```python
from build123d import *

# Parameters (mm, degrees)
F0_R     = 25
F1_DEPTH = 50
F2_R     = 25.5
F3_DEPTH = 10
F4_R     = 2
F5_R     = 1


with BuildPart() as f1:
    # F0 (on Top) → F1 (new body)
    with BuildSketch(Plane.XY):
        Circle(F0_R)
    extrude(amount=F1_DEPTH)

    # F2 (on face) → F3 (join)
    with BuildSketch(Plane.XY.offset(50)):
        Circle(F2_R)
    extrude(amount=F3_DEPTH)

    # F4
    f4_edges = [f1.edges().sort_by_distance(p)[0] for p in [
        (-25.5, 0, 60),
    ]]
    fillet(f4_edges, radius=F4_R)

    # F5
    f5_edges = [f1.edges().sort_by_distance(p)[0] for p in [
        (-25, 0, 0),
    ]]
    fillet(f5_edges, radius=F5_R)


solid = f1.part
```
The listing builds one solid part. Answer for the finished solid, in the listing's coordinates (mm). A direction names the side the tool comes from. Coordinates: 2 decimals unless noted, no trailing zeros. Write each loop counter-clockwise with the first axis right and the second up, starting at its lowest first coordinate (ties: lowest second). Pieces come first, ordered by that corner, then holes. Notation, with made-up numbers: (89.25, 55) - (99.25, 55) arc R22 ccw to (99.25, 70) - close; hole circle Ø5 at (85.5, 44.5). An arc over 180 degrees is marked (long way). Return JSON: item names as keys, results as strings. Group by question number.
Q1. The part is cut by section C-C on z = 33. Write down the section's boundary in (x, y), and give its area (3 significant figures).
Q2. Flat-ended cylindrical pins translate along their axes: pin 1 Ø10 at (x, z) = (13.5, 36) entering from +Y; pin 2 Ø10 at (x, z) = (13.5, 30) entering from -Y; pin 3 Ø4 at (y, z) = (7.5, 24.5) entering from -X. Find the tip coordinate at first contact, or state that the pin passes through.
Q3. The part is cut by section A-A on y = 0. Write down the section's boundary in (x, z).
Q4. Which of the six approach directions +Z, -Z, +X, -X, +Y, -Y give full straight-line access (tool end or side, diameter ignored) to faces 1 (the flat face through (0, 0, 60)), 2 (the flat face through (16.9, -18.8, 50))?
Q5. Find the intervals of material crossed by line 1 along X through (y, z) = (7, 47.5); line 2 along Y through (x, z) = (9.5, 26), in increasing order. Write a range as [from, to].
Evaluation:
{
 "1": {"outline": "circle Ø50 at (0, 0)", "area": "1,960 mm2"},
 "2": {"pin 1": "stops at y = 23.51", "pin 2": "stops at y = -23.51", "pin 3": "stops at x = -24.39"},
 "3": {"outline": "(-25.5, 50) - (-25, 50) - (-25, 1) arc R1 ccw to (-24, 0) - (24, 0) arc R1 ccw to (25, 1) - (25, 50) - (25.5, 50) - (25.5, 58) arc R2 ccw to (23.5, 60) - (-23.5, 60) arc R2 ccw to (-25.5, 58) - close"},
 "4": {"face 1": "+Z, +X, -X, +Y, -Y", "face 2": "-Z"},
 "5": {"line 1": "x = [-24, 24]", "line 2": "y = [-23.12, 23.12]"}
}
